```python
from build123d import *

# Parameters (mm, degrees)
F1_DEPTH = 80
F3_W     = 177
F3_H     = 70
F4_DEPTH = 5


# Not quite as in the source:
# - ends of sketch curves that miss each other by under 0.0002 mm in the source are joined


with BuildPart() as f1:
    # F0 (on Front) → F1 (new body)
    with BuildSketch(Plane.XZ):
        with BuildLine():
            Line((-220, 0), (0, 0))
            Line((0, 0), (220, 0))
            Line((220, 0), (220, 5.872634))
            ThreePointArc((220, 5.872634), (219.9686827703, 5.9800868873), (219.8845387701, 6.0538885071))
            ThreePointArc((219.8845387701, 6.0538885071), (169.4297421053, 23.1880267358), (116.462901, 28.9999923785))
            ThreePointArc((116.462901, 28.9999923785), (116.4045566452, 28.9913078859), (116.3512831377, 28.9659817952))
            ThreePointArc((116.3512831377, 28.9659817952), (105.4447272771, 23.7801763601), (93.5, 22))
            Line((93.5, 22), (93.5, 20))
            Line((93.5, 20), (0, 20))
            Line((0, 20), (-93.5, 20))
            Line((-93.5, 20), (-93.5, 22))
            ThreePointArc((-93.5, 22), (-105.4447272771, 23.7801763601), (-116.351282957, 28.965982064))
            ThreePointArc((-116.351282957, 28.965982064), (-116.4045566452, 28.9913078859), (-116.462901, 28.9999919938))
            ThreePointArc((-116.462901, 28.9999919938), (-169.4297421053, 23.1880267358), (-219.8845388425, 6.0538886623))
            ThreePointArc((-219.8845388425, 6.0538886623), (-219.9686827703, 5.9800868873), (-220, 5.872634))
            Line((-220, 5.872634), (-220, 0))
        make_face()
    extrude(amount=F1_DEPTH)

    # F3 (on face) → F4 (cut)
    with BuildSketch(Plane.XY.offset(20)):
        with Locations((0, -40)):
            Rectangle(F3_W, F3_H)
    extrude(amount=-F4_DEPTH, mode=Mode.SUBTRACT)


solid = f1.part
```
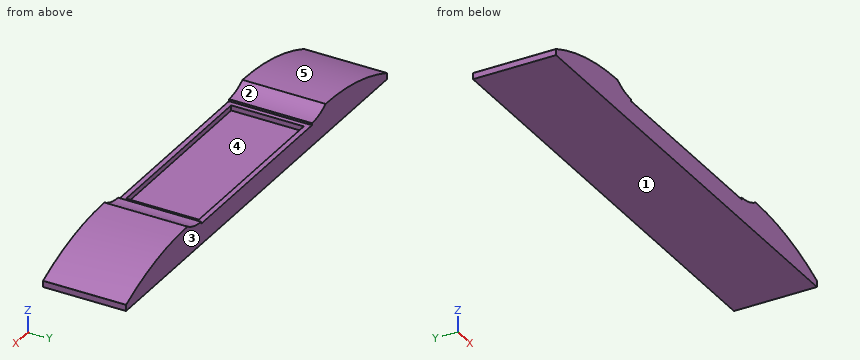
Can you work these out from the model? Positions are in its coordinate system, mm. Face numbers are marked on the shaded views. A direction names the side the tool comes from. Coordinates: 2 decimals unless noted, no trailing zeros. Order: outer loops, then holes, each group sorted by start corner. A loop starts at its lowest first (then second) coordinate and runs counter-clockwise, first axis right, second up.
1. Thinking about a two-plate mould opening in X: for the marked faces 3, 4 and 5, which applies, +X half, -X half, draft (parallel to the pull), parting line (faces both ways), or undercut?
2. I need wall thicknesses on line 1 (Z direction, x = 80, y = -5.5); line 2 (Z direction, x = 117, y = -15); line 3 (X direction, y = -41, z = 9). Which ranges of each line are inside material? Lowest first, please.
3. I'm going to push flat-ended pins straight in: pin 1 (24 mm diameter, centred on x = -13, y = -57.5, fed in from +Z); pin 2 (10 mm diameter, centred on x = -175, y = -72, fed in from +Z). Where does each tip first touch, or does it pass through?
4. If we section it at A-A (x = 81): Please give me the cut outline in (y, z), then the cut area to 3 significant figures.
5. For the marked faces 1 and 2, which set-ups out of +Z, -Z, +X, -X, +Y, -Y let a thin tool reach every point of the face, with its end or its side?
6. If we section it at C-C (x = -162): Please give me the cut outline in (y, z).
7. If we section it at B-B (y = -57): Please give me the cut outline in (x, z).
Entries:
1. face 3: draft
1. face 4: undercut
1. face 5: -X half
2. line 1: z = 0 to 15
2. line 2: z = 0 to 29
2. line 3: x = -213.32 to 213.32
3. pin 1: stops at z = 15
3. pin 2: stops at z = 23.06
4. outline: (-80, 0) - (0, 0) - (0, 20) - (-5, 20) - (-5, 15) - (-75, 15) - (-75, 20) - (-80, 20) - close
4. area: 1,250 mm2
5. face 1: -Z, +X, -X, +Y, -Y
5. face 2: +Z, +Y, -Y
6. outline: (-80, 0) - (0, 0) - (0, 24.72) - (-80, 24.72) - close
7. outline: (-220, 0) - (220, 0) - (220, 5.87) arc R0.2 ccw to (219.88, 6.05) arc R244.82 ccw to (116.46, 29) arc R0.2 ccw to (116.35, 28.97) arc R40.96 cw to (93.5, 22) - (93.5, 20) - (88.5, 20) - (88.5, 15) - (-88.5, 15) - (-88.5, 20) - (-93.5, 20) - (-93.5, 22) arc R40.96 cw to (-116.35, 28.97) arc R0.2 ccw to (-116.46, 29) arc R244.82 ccw to (-219.88, 6.05) arc R0.2 ccw to (-220, 5.87) - close
